For this review, take the finished solid that the model builds, in its own axes (mm). A direction names the side the tool comes from. Give positions to 0.01 mm unless a question says otherwise; leave off trailing zeros. Order: outer loops, then holes, each group sorted by start corner. A loop starts at its lowest first (then second) coordinate and runs counter-clockwise, first axis right, second up. Notation, with made-up numbers: (-29, 19) -> (13, 19) arc R14 ccw to (13, 45) -> close; hole circle Ø5 at (66.25, -33.5). An arc over 180 degrees is marked (long way). Return JSON: item names as keys, results as strings. Group by question number.
1) Add section C-C (x = 2.5). Give the boundary of the cut face in (y, z) (1 decimal), then the cut area to 3 significant figures.
2) Add section A-A (y = 0). Give the boundary of the cut face in (x, z), then the cut area to 3 significant figures.
3) To check wall thickness, follow line 1 along Y through (x, z) = (5, 0); line 2 along Z through (x, y) = (3.5, 27). State the ranges of each line that lie inside material, in increasing order.
4) Insertion check: P1, Ø2, axis at x = 7, z = -25.5, coming from the +Y side; P2, Ø2.5, axis at x = 4.5, z = 1.5, coming from the +Y side; P3, Ø2, axis at x = 6.5, y = -27, coming from the +Z side. Each pin has a flat end and moves straight along its axis. Give the tip position at first contact, or say it passes through.
5) For faces 1 (the face through (5, 4, 41)), 2 (the face through (5.1, 29.8, -30.3)), 3 (the face through (5, -41, -4)), 4 (the face through (5, -4, -41)), list the 3-axis set-ups (+Z, -Z, +X, -X, +Y, -Y) from which the entire face can be reached by the end or side of a thin tool; tool diameter is ignored.
6) The part is to be moulded in two halves that separate along Y. For faces 5 (the face through (5, 0, 39)), 6 (the face through (5, 4, -41)), 7 (the face through (5, 41, 4)), 8 (the face through (9.83, -29.18, -29.75)), say which applies: released by +Y, released by -Y, zero draft, split by the parting line, or undercut.
Autodesk Inventor part; units mm, degrees
ref_plane "Work Plane1" through (120.6234, 0, 0) normal (0, 1, 0) x (-1, 0, 0)
ref_plane "YZ Plane" through (0, 0, 0) normal (1, 0, 0) x (0, 1, 0)
ref_plane "XZ Plane" through (0, 0, 0) normal (0, 1, 0) x (-1, 0, 0)
sketch "草图1" plane through (0, 0, 0) normal (0, 0, 1) x (1, 0, 0)
  line L0 (0, 0) -> (10, 0)
  line L1 (0, 0) -> (0, 42.5)
  line L2 (0, 42.5) -> (10, 42.5)
  line L3 (10, 42.5) -> (10, 0)
  line L4 (0, 51) -> (0, -8.5)
  line L5 (-2, 0) -> (12, 0)
  dimension "d1" = 85
  dimension "d2" = 10
revolve "轴承体" add sketch "草图1" angle 360 about axis through (0, 0, 0) along (1, 0, 0)
sketch "草图2" plane through (0, 0, 0) normal (-1, 0, 0) x (0, 0, 1)
  circle A0 centre (0, 0) radius 42.5
  point P0 (0, 0)
hole "螺纹" at (0, 0, 0) direction (1, 0, 0) diameter 61.835 end through all
sketch "草图3" plane through (10, 0, 0) normal (1, 0, 0) x (0, 0, -1)
  circle A0 centre (0, 0) radius 42.5
  line L0 (-4, 42.3113) -> (-4, 39)
  line L1 (-4, 39) -> (4, 39)
  line L2 (4, 39) -> (4, 42.3113)
  line L3 (0, -59.5) -> (0, 59.5)
  line L4 (-59.5, 0) -> (59.5, 0)
  dimension "d12" = 4
  dimension "d13" = 4
  dimension "d14" = 39
extrude "沟槽1" cut sketch "草图3" against normal through all contours L2 L1 L3 A0 | L3 L1 L0 A0
pattern_circular "IDS_ARRAYGROOVE{1}" count 4 over 360 about axis through (-10, 0, 0) along (1, 0, 0) of "沟槽1"
chamfer "倒角1" distance 1 angle 45 4 edges at (0, 30.052, -30.052) (0, 30.052, 30.052) (0, -30.052, -30.052) (0, -30.052, 30.052) measured on face at (0, -20.4276, -32.5865)
chamfer "倒角2" distance 1 angle 45 4 edges at (10, 30.052, 30.052) (10, 30.052, -30.052) (10, -30.052, -30.052) (10, -30.052, 30.052) measured on face at (10, -20.4276, -32.5865)
chamfer "倒角3" distance 1.6 angle 30 1 edges at (10, 0, -30.9175) measured on face at (10, 20.075, -32.0252)
chamfer "倒角4" distance 1.6 angle 30 1 edges at (0, 0, -30.9175) measured on face at (0, -20.075, -32.0252)
ref_plane "Work Plane1" through (120.6234, 0, 0) normal (0, 1, 0) x (-1, 0, 0)
equation "\"d1\" = SD2"
equation "\"d2\" = KOH"
equation "\"d12\" = 0.5 * SNB"
equation "\"d13\" = 0.5 * SNB"
equation "\"d14\" = 0.5 * SD2 - SNT"
equation "\"d10\" = -0.5 * LADI + 0.5 * SD2"
equation "\"d11\" = FAWI"
equation "\"d41\" = -0.5 * LADI + 0.5 * SD2"
equation "\"d25\" = -0.5 * LADI + 0.5 * SD2"
equation "\"d27\" = FAWI"
equation "\"d42\" = -0.5 * LADI + 0.5 * SD2"
equation "\"d18\" = 0.025 * NND"
equation "\"d43\" = 0.025 * NND"
equation "\"d20\" = 0.025 * NND"
equation "\"d44\" = 0.025 * NND"
equation "\"NND\" = 64"
equation "\"KOH\" = 10"
equation "\"SD2\" = 85"
equation "\"SNB\" = 8"
equation "\"SNT\" = 3.5"
equation "\"LADI\" = 83"
equation "\"FAWI\" = 45deg"
equation "\"GUL\" = 0.61345 * PTC"
equation "\"PHH\" = 1"
equation "\"THREADDIA\" = 64"
equation "\"TOA\" = 30deg"
equation "\"PTC\" = 2"
equation "\"FAWI1\" = 60deg"
equation "\"GAL\" = 0.61345 * PTC"
equation "\"GD1\" = THREADDIA - 1.2269 * PTC"
properties part number "螺母 GB 810 M64 x 2" material "钢，软"
Evaluation:
{
 "1": {"outline": "(-42.3, -4) arc R42.5 ccw to (-4, -42.3) -> (-4, -39) -> (4, -39) -> (4, -42.3) arc R42.5 ccw to (42.3, -4) -> (39, -4) -> (39, 4) -> (42.3, 4) arc R42.5 ccw to (4, 42.3) -> (4, 39) -> (-4, 39) -> (-4, 42.3) arc R42.5 ccw to (-42.3, 4) -> (-39, 4) -> (-39, -4) -> close; hole circle Ø61.8 at (0, 0)", "area": "2,560 mm^2"},
 "2": {"outline": "(0, -39) -> (10, -39) -> (10, -32.52) -> (9.08, -30.92) -> (0.92, -30.92) -> (0, -32.52) -> close; (0, 32.52) -> (0.92, 30.92) -> (9.08, 30.92) -> (10, 32.52) -> (10, 39) -> (0, 39) -> close", "area": "159 mm^2"},
 "3": {"line 1": "-39 to -30.92, 30.92 to 39", "line 2": "-32.82 to -15.06, 15.06 to 32.82"},
 "4": {"P1": "y = 34.73", "P2": "y = 39", "P3": "z = 33.62"},
 "5": {"face 1": "+Z, +X, -X", "face 2": "-Z, +X, -X, +Y", "face 3": "+X, -X, -Y", "face 4": "-Z, +X, -X"},
 "6": {"face 5": "undercut", "face 6": "undercut", "face 7": "zero draft", "face 8": "released by -Y"}
}
